Input: part model. Units: mm. Frame: model coordinates. Face numbers are marked on the shaded views. Round coordinates to 2 decimals unless told otherwise and drop trailing zeros. Loops run counter-clockwise (first coordinate to the right, second up) from the corner with the lowest first, then second, coordinate; pieces in that order, holes last. Notation, with made-up numbers: (-39, 3.25) - (9, 3.25) arc R24 cw to (9, 39.25) - close; hole circle Ø11 at (32.25, 68). An arc over 180 degrees is marked (long way). Use CSV: the item, a comma, the result in double quotes. Start each with the question number.
1. Pin query (flat end, axial travel): P1, Ø1, axis at x = -72.5, y = 39, coming from the +Z side; P2, Ø4, axis at x = -69.5, y = -9, coming from the +Z side; P3, Ø3, axis at y = -42, z = 39.5, coming from the -X side. Return the tip coordinate at first contact, or that it passes through.
2. Cut plane B-B (z = 54.5). Return loops of the section in (x, y), and give its area (3 significant figures).
3. Cut plane D-D (x = 95). Return loops of the section in (y, z), and give its area (3 significant figures).
4. Cut plane C-C (y = -17). Return loops of the section in (x, z), and give its area (3 significant figures).
5. Pull-direction query (X, two-part tool) for the marked faces 1, 2, 3 and 4; classes: +X half, -X half, draft (parallel to the pull), parting line (faces both ways), or undercut.
6. Cut plane A-A (x = -3.5). Return loops of the section in (y, z), and give its area (3 significant figures).
7. Material intervals for probe 1 along X at (y, z) = (-18.5, 3); probe 2 along X at (y, z) = (-32, 48); probe 3 along Y at (x, z) = (-95, 51.75), sorted ascending. Write a range as from..to.
```python
from build123d import *

# Parameters (mm, degrees)
SKETCH_W                      = 200
SKETCH_H                      = 75
PAD_DEPTH                     = 60
POCKET_DEPTH                  = 58
SKETCH002_R                   = 2.5
POCKET001_DEPTH               = 15
SKETCH002_MIRRORED_2_R        = 2.5
POCKET001_MIRRORED_2_DEPTH    = 15
PAD001_DEPTH                  = 10
PAD001_MIRRORED002_2_DEPTH    = 10
SKETCH004_R                   = 1.5
POCKET002_DEPTH               = 10
SKETCH004_MIRRORED004_2_R     = 1.5
POCKET002_MIRRORED004_2_DEPTH = 10


with BuildPart() as part:
    # Sketch (on DatumPlane) → Pad (new body)
    with BuildSketch(Plane.XY):
        Rectangle(SKETCH_W, SKETCH_H)
    extrude(amount=PAD_DEPTH)

    # Sketch001 (on DatumPlane) → Pocket (cut)
    with BuildSketch(Plane.XY.offset(60)):
        Polygon((-97.5, -23), (-97.5, 23), (-85.5, 35), (85.5, 35), (97.5, 23), (97.5, -23), (85.5, -35), (-85.5, -35), align=None)
    extrude(amount=-POCKET_DEPTH, mode=Mode.SUBTRACT)

    # Sketch002 (on DatumPlane) → Pocket001 (cut)
    with BuildSketch(Plane.XY.offset(60)):
        with Locations((-95, 32.5)):
            Circle(SKETCH002_R)
    pocket001 = extrude(amount=-POCKET001_DEPTH, mode=Mode.SUBTRACT)

    # Sketch002 Mirrored 2 → Pocket001 Mirrored 2 (cut)
    with BuildSketch(Plane(origin=(0, 0, 60), x_dir=(-1, 0, 0), z_dir=(0, 0, -1))):
        with Locations((-95, 32.5)):
            Circle(SKETCH002_MIRRORED_2_R)
    pocket001_mirrored_2 = extrude(amount=POCKET001_MIRRORED_2_DEPTH, mode=Mode.SUBTRACT)

    # Mirrored001: Pocket001, Pocket001 Mirrored 2 across XZ
    add(pocket001.mirror(Plane.XZ), mode=Mode.SUBTRACT)
    add(pocket001_mirrored_2.mirror(Plane.XZ), mode=Mode.SUBTRACT)

    # Sketch003 (on DatumPlane) → Pad001 (join, symmetric)
    with BuildSketch(Plane.YZ.offset(-75)):
        with BuildLine():
            Line((41, 43), (37.5, 43))
            Line((37.5, 43), (37.5, 37))
            Line((37.5, 37), (41, 37))
            ThreePointArc((41, 37), (44, 40), (41, 43))
        make_face()
        with BuildLine():
            Line((41, 7), (37.5, 7))
            Line((37.5, 7), (37.5, 13))
            Line((37.5, 13), (41, 13))
            ThreePointArc((41, 7), (44, 10), (41, 13))
        make_face()
    pad001 = extrude(amount=PAD001_DEPTH, both=True)

    # Sketch003 Mirrored002 2 → Pad001 Mirrored002 2 (add, symmetric)
    with BuildSketch(Plane.YZ.offset(75)):
        with BuildLine():
            Line((41, 43), (37.5, 43))
            Line((37.5, 43), (37.5, 37))
            Line((37.5, 37), (41, 37))
            ThreePointArc((41, 37), (44, 40), (41, 43))
        make_face()
        with BuildLine():
            Line((41, 7), (37.5, 7))
            Line((37.5, 7), (37.5, 13))
            Line((37.5, 13), (41, 13))
            ThreePointArc((41, 7), (44, 10), (41, 13))
        make_face()
    pad001_mirrored002_2 = extrude(amount=-PAD001_MIRRORED002_2_DEPTH, both=True)

    # Mirrored003: Pad001, Pad001 Mirrored002 2 across XZ
    add(pad001.mirror(Plane.XZ))
    add(pad001_mirrored002_2.mirror(Plane.XZ))

    # Sketch004 (on DatumPlane) → Pocket002 (cut, symmetric)
    with BuildSketch(Plane.YZ.offset(-75)):
        with Locations((41.5, 40)):
            Circle(SKETCH004_R)
        with Locations((41.5, 10)):
            Circle(SKETCH004_R)
    pocket002 = extrude(amount=POCKET002_DEPTH, both=True, mode=Mode.SUBTRACT)

    # Sketch004 Mirrored004 2 → Pocket002 Mirrored004 2 (cut, symmetric)
    with BuildSketch(Plane.YZ.offset(75)):
        with Locations((41.5, 40)):
            Circle(SKETCH004_MIRRORED004_2_R)
        with Locations((41.5, 10)):
            Circle(SKETCH004_MIRRORED004_2_R)
    pocket002_mirrored004_2 = extrude(amount=-POCKET002_MIRRORED004_2_DEPTH, both=True, mode=Mode.SUBTRACT)

    # Mirrored005: Pocket002, Pocket002 Mirrored004 2 across XZ
    add(pocket002.mirror(Plane.XZ), mode=Mode.SUBTRACT)
    add(pocket002_mirrored004_2.mirror(Plane.XZ), mode=Mode.SUBTRACT)


solid = part.part
```
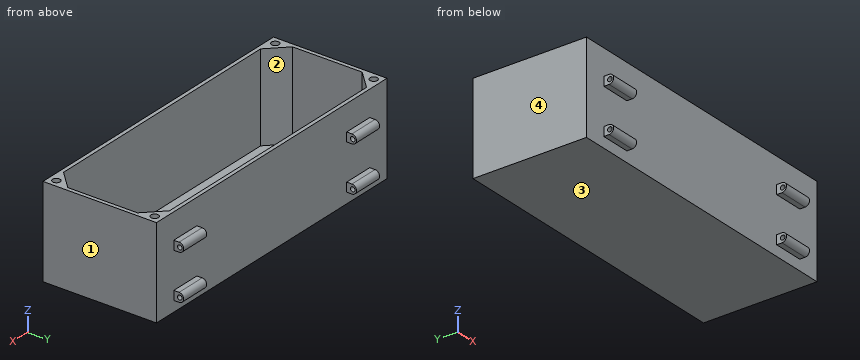
Established:
1,P1,"stops at z = 43"
1,P2,"stops at z = 2"
1,P3,"stops at x = -85"
2,outline,"(-100, -37.5) - (100, -37.5) - (100, 37.5) - (-100, 37.5) - close; hole circle Ø5 at (-95, -32.5); hole (-97.5, -23) - (-85.5, -35) - (85.5, -35) - (97.5, -23) - (97.5, 23) - (85.5, 35) - (-85.5, 35) - (-97.5, 23) - close; hole circle Ø5 at (-95, 32.5); hole circle Ø5 at (95, -32.5); hole circle Ø5 at (95, 32.5)"
2,area,"1,560 mm2"
3,outline,"(-37.5, 0) - (37.5, 0) - (37.5, 60) - (35, 60) - (35, 45) - (30, 45) - (30, 60) - (25.5, 60) - (25.5, 2) - (-25.5, 2) - (-25.5, 60) - (-30, 60) - (-30, 45) - (-35, 45) - (-35, 60) - (-37.5, 60) - close"
3,area,"1,390 mm2"
4,outline,"(-100, 0) - (100, 0) - (100, 60) - (97.5, 60) - (97.5, 2) - (-97.5, 2) - (-97.5, 60) - (-100, 60) - close"
4,area,"690 mm2"
5,face 1,"+X half"
5,face 2,"undercut"
5,face 3,"draft"
5,face 4,"-X half"
6,outline,"(-37.5, 0) - (37.5, 0) - (37.5, 60) - (35, 60) - (35, 2) - (-35, 2) - (-35, 60) - (-37.5, 60) - close"
6,area,"440 mm2"
7,probe 1,"x = -100..-97.5, 97.5..100"
7,probe 2,"x = -100..-97.45, -92.55..-88.5, 88.5..92.55, 97.45..100"
7,probe 3,"y = -37.5..-35, -30..-25.5, 25.5..30, 35..37.5"
